The figure shows three views and two pictorial views of one solid part (mm, origin at its lowest corner). Answer the questions. A direction names the side the tool comes from. Give positions to 0.01 mm unless a question says otherwise; leave off trailing zeros. Write each loop counter-clockwise with the first axis right and the second up, starting at its lowest first coordinate (ties: lowest second). Pieces come first, ordered by that corner, then holes. Notation, with made-up numbers: (71, -13) -> (129, -13) arc R19 ccw to (129, 3) -> close; hole circle Ø2 at (70.5, 46.5). An arc over 180 degrees is marked (long way). Answer as CSV lines item,"result". Start each with the question number.
1. Find the intervals of material crossed by line 1 (Z direction, x = 1.25, y = 3.25) (1 decimal); line 2 (Y direction, x = 17.75, z = 4.75); line 3 (X direction, y = 0.5, z = 1.75), in increasing order.
2. The part is cut by section B-B, the plane y = 7.5. Determine the outline of the cut face in (x, z) (1 decimal).
3. The part is cut by section C-C, the plane z = 2.25. Give the number of separate pieces and of enclosed holes in the cut face, and give its area (3 significant figures).
4. For a pull along X with two mould halves and no side action, classify the marked faces 1, 2 and 3 as pulls with the +X half, pulls with the -X half, needs draft (parallel to the pull), parting line crosses it, or undercut.
5. The part is cut by section A-A, the plane x = 6. Determine the outline of the cut face in (y, z) (1 decimal), and give its area (3 significant figures).
6. A tool of negligible diameter and unlimited length cuts with its end or side. For the marked faces 4, 5 and 6, from which of +Z, -Z, +X, -X, +Y, -Y can it reach the whole face along a straight path? Write none if from no direction.
7. The part is cut by section D-D, the plane x = 16.75. Determine the outline of the cut face in (y, z) (1 decimal).
8. Given pin 1 (1.5 mm diameter, centred on x = 14, z = 6, fed in from +Y); pin 2 (0.6 mm diameter, centred on x = 24, z = 2, fed in from +Y); pin 3 (0.8 mm diameter, centred on y = 0.5, z = 2, fed in from +X); pin 4 (1.7 mm diameter, centred on x = 6.41, y = 5.04, fed in from +Z) (3 decimals), each flat-ended and moving along its own axis, determine where each tip first touches the part or whether it passes through.
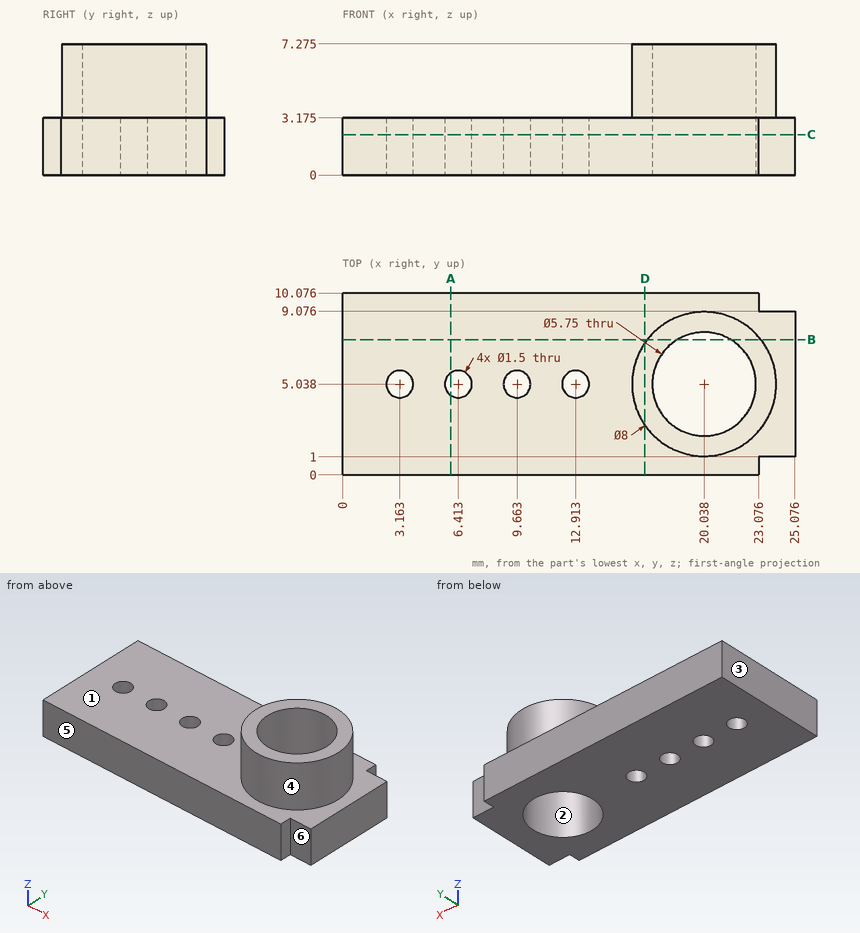
Results found:
1,line 1,"z = 0 to 3.2"
1,line 2,"y = 1.76 to 3.3, 6.78 to 8.32"
1,line 3,"x = 0 to 23.08"
2,outline,"(0, 0) -> (18.6, 0) -> (18.6, 7.3) -> (16.9, 7.3) -> (16.9, 3.2) -> (0, 3.2) -> close; (21.5, 0) -> (25.1, 0) -> (25.1, 3.2) -> (23.2, 3.2) -> (23.2, 7.3) -> (21.5, 7.3) -> close"
3,separate pieces,"1"
3,enclosed holes,"5"
3,area,"216 mm²"
4,face 1,"needs draft"
4,face 2,"undercut"
4,face 3,"pulls with the -X half"
5,outline,"(0, 0) -> (4.4, 0) -> (4.4, 3.2) -> (0, 3.2) -> close; (5.7, 0) -> (10.1, 0) -> (10.1, 3.2) -> (5.7, 3.2) -> close"
5,area,"28.0 mm²"
6,face 4,"+Z"
6,face 5,"+Z, -Z, +X, -X, -Y"
6,face 6,"+Z, -Z, +X, -Y"
7,outline,"(0, 0) -> (10.1, 0) -> (10.1, 3.2) -> (7.3, 3.2) -> (7.3, 7.3) -> (2.8, 7.3) -> (2.8, 3.2) -> (0, 3.2) -> close"
8,pin 1,"passes through"
8,pin 2,"stops at y = 9.08"
8,pin 3,"stops at x = 23.08"
8,pin 4,"stops at z = 3.175"
